Geometry check sheet. Reference: the model listing, model coordinates, mm. Face numbers are marked on the shaded views. A direction names the side the tool comes from. Give positions to 0.01 mm unless a question says otherwise; leave off trailing zeros. Order: outer loops, then holes, each group sorted by start corner. A loop starts at its lowest first (then second) coordinate and runs counter-clockwise, first axis right, second up. Notation, with made-up numbers: M 16.5,35 L 30.5,35 A21 ccw 30.5,61 Z; hole C -34.5,-14.5 d8. An arc over 180 degrees is marked long. Use CSV: the item, a comma, the result in double quotes. Start each with the question number.
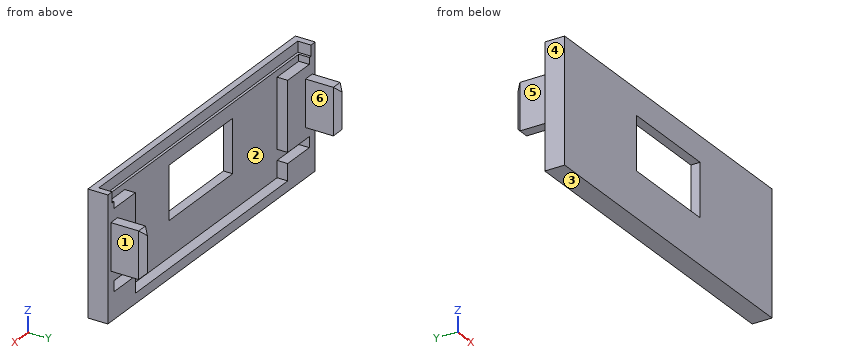
from build123d import *

# Parameters (mm, degrees)
ESQUISSE1_W                  = 49
ESQUISSE1_H                  = 3
BOSS_EXTRU_1_DEPTH           = 18.6
ENL_V_MAT_EXTRU_2_DEPTH      = 1.6
ENL_V_MAT_EXTRU_3_REACH      = 32.802
ESQUISSE6_W                  = 15
ESQUISSE6_H                  = 8
ESQUISSE7_W                  = 1.6
ESQUISSE7_H                  = 7
BOSS_EXTRU_2_DEPTH           = 5
CHANFREIN1_SIZE              = 0.8
CHANFREIN1_OF_SYM_TRIE1_SIZE = 0.8
ESQUISSE8_W                  = 47
ESQUISSE8_H                  = 2
ENL_V_MAT_EXTRU_4_DEPTH      = 1.6


with BuildPart() as part:
    # Esquisse1 → Boss.-Extru.1 (new body)
    with BuildSketch(Plane.XY):
        Rectangle(ESQUISSE1_W, ESQUISSE1_H)
    extrude(amount=BOSS_EXTRU_1_DEPTH)

    # Esquisse5 → Enlèv. mat.-Extru.2 (cut)
    with BuildSketch(Plane(origin=(0, 1.5, 0), x_dir=(1, 0, 0), z_dir=(0, 1, 0))):
        Polygon((-23.1, -4), (-23.1, -5.6), (-18, -5.6), (-18, -16), (-23.1, -16), (-23.1, -17.6), (23.1, -17.6), (23.1, -16), (18, -16), (18, -5.6), (23.1, -5.6), (23.1, -4), (18, -4), (18, -1.5), (-18, -1.5), (-18, -4), align=None)
    extrude(amount=-ENL_V_MAT_EXTRU_2_DEPTH, mode=Mode.SUBTRACT)

    # Esquisse6 → Enlèv. mat.-Extru.3 (cut, up to next)
    with BuildSketch(Plane(origin=(0, -0.1, 0), x_dir=(1, 0, 0), z_dir=(0, 1, 0)), mode=Mode.PRIVATE) as enl_v_mat_extru_3_sk1:
        with Locations((0, -10.8)):
            Rectangle(ESQUISSE6_W, ESQUISSE6_H)
    enl_v_mat_extru_3_tool1 = extrude(enl_v_mat_extru_3_sk1.sketch, amount=-ENL_V_MAT_EXTRU_3_REACH, mode=Mode.PRIVATE) & part.part
    add(enl_v_mat_extru_3_tool1.solids().sort_by_distance((0, -0.1, 10.8))[0], mode=Mode.SUBTRACT)

    # Esquisse7 → Boss.-Extru.2 (add)
    with BuildSketch(Plane(origin=(0, 1.5, 0), x_dir=(1, 0, 0), z_dir=(0, 1, 0))):
        with Locations((-23, -10.8)):
            Rectangle(ESQUISSE7_W, ESQUISSE7_H)
    boss_extru_2 = extrude(amount=BOSS_EXTRU_2_DEPTH)

    # Chanfrein1
    chanfrein1_edges = [part.edges().sort_by_distance(p)[0] for p in [
        (-22.2, 6.5, 10.8),
        (-23, 6.5, 7.3),
        (-23.8, 6.5, 10.8),
        (-23, 6.5, 14.3),
    ]]
    chamfer(chanfrein1_edges, length=CHANFREIN1_SIZE - 0.0001)  # a hair under: the kernel refuses the full size

    # Symétrie1: Boss.-Extru.2 across plane
    add(boss_extru_2.mirror(Plane(origin=(0, 0, 0), x_dir=(0, 0, 1), z_dir=(1, 0, 0))))

    # Chanfrein1 of Symétrie1
    chanfrein1_of_sym_trie1_edges = [part.edges().sort_by_distance(p)[0] for p in [
        (22.2, 6.5, 10.8),
        (23, 6.5, 7.3),
        (23.8, 6.5, 10.8),
        (23, 6.5, 14.3),
    ]]
    chamfer(chanfrein1_of_sym_trie1_edges, length=CHANFREIN1_OF_SYM_TRIE1_SIZE - 0.0001)  # a hair under: the kernel refuses the full size

    # Esquisse8 → Enlèv. mat.-Extru.4 (cut)
    with BuildSketch(Plane.XY.offset(18.6)):
        with Locations((0, 0.5)):
            Rectangle(ESQUISSE8_W, ESQUISSE8_H)
    extrude(amount=-ENL_V_MAT_EXTRU_4_DEPTH, mode=Mode.SUBTRACT)


solid = part.part
(1) Draft check along X on the marked faces 1, 2 and 3. Enter one of: +X half, -X half, draft (parallel to the pull), parting line (faces both ways), or undercut.
(2) Sectioned sample at B-B on x = -7. Record the cut outline in (y, z), then the cut area to 3 significant figures.
(3) Go/stop test with flat-tipped pins: P1, Ø2, axis at y = 4, z = 9.5, coming from the -X side; P2, Ø0.8, axis at x = 23, y = 4.5, coming from the -Z side; P3, Ø1.3, axis at x = -23, y = 3.5, coming from the +Z side. Record where each tip stops, or that it passes through.
(4) Thickness scan on line 1 (X direction, y = 1.25, z = 9.5); line 2 (X direction, y = 4, z = 9.5); line 3 (Y direction, x = 5.5, z = 5). Record the ranges inside material, lowest first.
(5) Sectioned sample at A-A on y = 3.75. Record the cut outline in (x, z).
(6) Access from +Z, -Z, +X, -X, +Y, -Y to the whole of each face (thin tool, end or side, straight path). Record for the marked faces 4, 5 and 6.
(7) Sectioned sample at C-C on y = -1. Record the cut outline in (x, z), then the cut area to 3 significant figures.
Responses:
1,face 1,"+X half"
1,face 2,"undercut"
1,face 3,"draft"
2,outline,"M -1.5,0 L 1.5,0 L 1.5,1.5 L -0.1,1.5 L -0.1,6.8 L -1.5,6.8 Z; M -1.5,14.8 L -0.1,14.8 L -0.1,17 L -0.5,17 L -0.5,18.6 L -1.5,18.6 Z"
2,area,"16.6 mm2"
3,P1,"x = -23.8"
3,P2,"z = 7.3"
3,P3,"z = 14.3"
4,line 1,"-24.5 to -18, 18 to 24.5"
4,line 2,"-23.8 to -22.2, 22.2 to 23.8"
4,line 3,"-1.5 to -0.1"
5,outline,"M -23.8,7.3 L -22.2,7.3 L -22.2,14.3 L -23.8,14.3 Z; M 22.2,7.3 L 23.8,7.3 L 23.8,14.3 L 22.2,14.3 Z"
6,face 4,"+Z, -Z, -X, +Y, -Y"
6,face 5,"+Z, -Z, -X, +Y"
6,face 6,"+Z, -Z, +Y"
7,outline,"M -24.5,0 L 24.5,0 L 24.5,18.6 L -24.5,18.6 Z; hole M -7.5,6.8 L 7.5,6.8 L 7.5,14.8 L -7.5,14.8 Z"
7,area,"791 mm2"
